from build123d import *

# Parameters (mm, degrees)
F0_R        = 2.35
F1_DEPTH    = 11.43
F0_R_2      = 4.636
F2_DEPTH    = 3.81
F0_R_3      = 11
F3_DEPTH    = 2.54
F5_DEPTH    = 1.27
F6_T1_DEPTH = 12.7
F6_T3_DEPTH = 7.62
F6_T5_DEPTH = 4.445
F6_T7_DEPTH = 4.079017898
F6_T9_DEPTH = 6.0188206533


# Not quite as in the source:
# - a fillet or chamfer that OpenCascade refuses, or shapes differently, is made with other operations: its cross-section is extruded or revolved along the edge and cut away or added


with BuildPart() as f1:
    # F0 (on Top) → F1 (new body)
    with BuildSketch(Plane.XY):
        Circle(F0_R)
    extrude(amount=F1_DEPTH)

    # F0 (on Top) → F2 (join)
    with BuildSketch(Plane.XY):
        Circle(F0_R_2)
        Circle(F0_R, mode=Mode.SUBTRACT)
    extrude(amount=F2_DEPTH)

    # F0 (on Top) → F3 (join)
    with BuildSketch(Plane.XY):
        Circle(F0_R_3)
        Circle(F0_R_2, mode=Mode.SUBTRACT)
    extrude(amount=F3_DEPTH)

    # F4 (on face) → F5 (join)
    with BuildSketch(Plane.XY):
        with BuildLine():
            ThreePointArc((0, -6.7733326328), (-6.1696334492, -0.6777773574), (0, 5.417777918))
            ThreePointArc((0, 5.417777918), (1.9417265012, 4.2834880284), (2.4694073737, 2.0975172472))
            Line((2.4694073737, 2.0975172472), (4.8922184175, 2.0975172472))
            ThreePointArc((4.8922184175, 2.0975172472), (3.5875761059, 5.9808584475), (0, 7.9586673672))
            ThreePointArc((0, 7.9586673672), (-8.382, -0.4233326328), (0, -8.8053326328))
            ThreePointArc((0, -8.8053326328), (3.39954986, -7.3527295439), (5.0117596984, -4.0259030648))
            Line((5.0117596984, -4.0259030648), (2.4717596984, -4.0259030648))
            ThreePointArc((2.4717596984, -4.0259030648), (1.8244333866, -5.9291174694), (0, -6.7733326328))
        make_face()
        with BuildLine():
            Line((4.8922184175, 2.0975172472), (2.4694073737, 2.0975172472))
            ThreePointArc((2.4694073737, 2.0975172472), (2.3960471942, 1.7747190007), (2.2859995271, 1.4625172472))
            Line((2.2859995271, 1.4625172472), (4.8259995271, 1.4625172472))
            ThreePointArc((4.8259995271, 1.4625172472), (4.8680955625, 1.7790801102), (4.8922184175, 2.0975172472))
        make_face()
        with BuildLine():
            ThreePointArc((2.2859995271, 1.4625172472), (2.3960471942, 1.7747190007), (2.4694073737, 2.0975172472))
            Line((2.4694073737, 2.0975172472), (0.3809995271, 2.0975172472))
            Line((0.3809995271, 2.0975172472), (0.3809995271, 0.8275172472))
            Line((0.3809995271, 0.8275172472), (6.7309995271, 0.8275172472))
            Line((6.7309995271, 0.8275172472), (6.7309995271, 2.0975172472))
            Line((6.7309995271, 2.0975172472), (4.8922184175, 2.0975172472))
            ThreePointArc((4.8922184175, 2.0975172472), (4.8680955625, 1.7790801102), (4.8259995271, 1.4625172472))
            Line((4.8259995271, 1.4625172472), (2.2859995271, 1.4625172472))
        make_face()
    extrude(amount=-F5_DEPTH)

    # F6: fillet of radius 1.27 on 5 edges, made by hand

    # F6_s2 → F6_t1 (cut)
    with BuildSketch(Plane.YZ.offset(-2.7940004729)):
        with BuildLine():
            ThreePointArc((0.8275172472, 0), (1.1994916351, -0.8980256121), (2.0975172472, -1.27))
            Line((2.0975172472, -1.27), (0.8275172472, -1.27))
            Line((0.8275172472, -1.27), (0.8275172472, 0))
        make_face()
    extrude(amount=F6_T1_DEPTH, mode=Mode.SUBTRACT)

    # F6_s4 → F6_t3 (cut)
    with BuildSketch(Plane.XZ.offset(-5.2725172472)):
        with BuildLine():
            ThreePointArc((6.7309995271, 0), (6.3590251392, -0.8980256121), (5.4609995271, -1.27))
            Line((5.4609995271, -1.27), (6.7309995271, -1.27))
            Line((6.7309995271, -1.27), (6.7309995271, 0))
        make_face()
    extrude(amount=F6_T3_DEPTH, mode=Mode.SUBTRACT)

    # F6_s6 → F6_t5 (cut)
    with BuildSketch(Plane.XZ.offset(-2.0975172472)):
        with BuildLine():
            ThreePointArc((0.3809995271, 0), (0.752973915, -0.8980256121), (1.6509995271, -1.27))
            Line((1.6509995271, -1.27), (0.3809995271, -1.27))
            Line((0.3809995271, -1.27), (0.3809995271, 0))
        make_face()
    extrude(amount=F6_T5_DEPTH, mode=Mode.SUBTRACT)

    # F6_s8 → F6_t7 (cut)
    with BuildSketch(Plane.XY.offset(-4.079017898)):
        with BuildLine():
            ThreePointArc((3.5953668576, -4.0259030648), (2.8338642738, -4.2795301928), (2.3765155692, -4.9391096556))
            ThreePointArc((2.3765155692, -4.9391096556), (2.4655394537, -4.4868244195), (2.4717596984, -4.0259030648))
            Line((2.4717596984, -4.0259030648), (3.5953668576, -4.0259030648))
        make_face()
    extrude(amount=F6_T7_DEPTH, mode=Mode.SUBTRACT)

    # F6_s10 → F6_t9 (cut)
    with BuildSketch(Plane.XY.offset(-6.0188206533)):
        with BuildLine():
            ThreePointArc((4.4971207542, -5.8543872382), (4.4340465678, -4.6237330343), (3.3565088886, -4.0259030648))
            Line((3.3565088886, -4.0259030648), (5.0117596984, -4.0259030648))
            ThreePointArc((5.0117596984, -4.0259030648), (4.837388646, -4.9634915319), (4.4971207542, -5.8543872382))
        make_face()
    extrude(amount=F6_T9_DEPTH, mode=Mode.SUBTRACT)


solid = f1.part
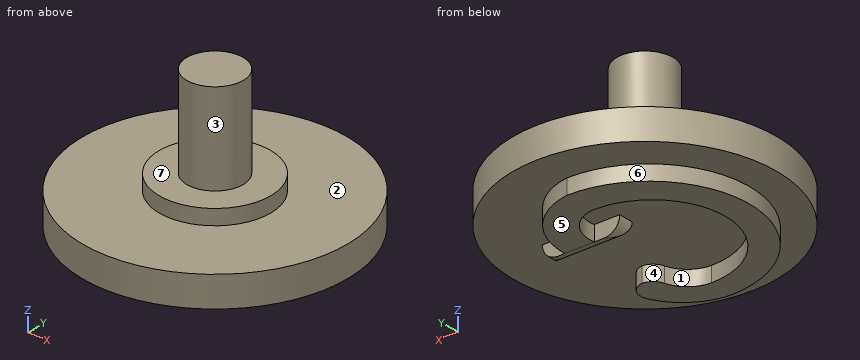
Could you check a few things on this model? Use its own coordinates, in mm. Face numbers are marked on the shaded views. A direction names the side the tool comes from. Give positions to 0.01 mm unless a question says otherwise; leave off trailing zeros. Loops run counter-clockwise (first coordinate to the right, second up) from the corner with the lowest first, then second, coordinate; pieces in that order, holes last. Notation, with made-up numbers: M -14.5,45.25 L -2.5,45.25 A11 cw -2.5,49.25 Z; hole C 62.5,55 d9. An arc over 180 degrees is marked long. Answer as a JSON object with one key per item and string values.
Q1. For the marked faces 4, 5, 6 and 7, which set-ups out of +Z, -Z, +X, -X, +Y, -Y let a thin tool reach every point of the face, with its end or its side?
Values found:
{"face 4": "-Z", "face 5": "-Z, +X, -X, +Y, -Y", "face 6": "-Z, -X", "face 7": "+Z"}
Q2. Suppose I cut it at A-A, the plane y = -7.5. List the corners of the cut face in (x, z) for me, plus the area to 3 significant figures.
Values found:
{"outline": "M -8.05,0 L -4.49,0 L -4.49,-1.27 L 3.24,-1.27 L 3.24,0 L 8.05,0 L 8.05,2.54 L -8.05,2.54 Z", "area": "50.7 mm²"}
Q3. Suppose I cut it at D-D, the plane y = 0. List the corners of the cut face in (x, z) for me, plus the area to 3 significant figures.
Values found:
{"outline": "M -11,0 L -8.37,0 L -8.37,-1.27 L -6.13,-1.27 L -6.13,0 L 11,0 L 11,2.54 L 4.64,2.54 L 4.64,3.81 L 2.35,3.81 L 2.35,11.43 L -2.35,11.43 L -2.35,3.81 L -4.64,3.81 L -4.64,2.54 L -11,2.54 Z", "area": "106 mm²"}
Q4. If we mould it in two halves opening along X, with no side actions, what happens to the marked faces 1, 2 and 3? For each: pulls with the +X half, pulls with the -X half, needs draft (parallel to the pull), parting line crosses it, or undercut.
Values found:
{"face 1": "undercut", "face 2": "needs draft", "face 3": "parting line crosses it"}
Q5. If I drill on probe 1 along Z at (x, y) = (-5.5, 7.75); probe 2 along Z at (x, y) = (-4.25, 5.5); probe 3 along X at (y, z) = (-9.5, 0.5), over which ranges is the centre line in solid material (lowest first)? Write a range as [from, to].
Values found:
{"probe 1": "z = [0, 2.54]", "probe 2": "z = [-1.27, 2.54]", "probe 3": "x = [-5.55, 5.55]"}
Q6. Suppose I cut it at C-C, the plane z = 7.75. List the corners of the cut face in (x, y) for me, plus the area to 3 significant figures.
Values found:
{"outline": "C 0,0 d4.7", "area": "17.3 mm²"}
Q7. For P1, Ø0.6, axis at x = 1, z = -0.5, coming from the +Y side; P2, Ø1.5, axis at x = -2.5, z = 0.5, coming from the +Y side; P3, Ø3, axis at x = -6.5, y = -0.5, coming from the +Z side, each with a flat end and sliding along its axis, tell me the tip position at first contact or that it passes through.
Values found:
{"P1": "stops at y = 7.82", "P2": "stops at y = 10.86", "P3": "stops at z = 2.54"}
Q8. Suppose I cut it at B-B, the plane x = -6.5. List the corners of the cut face in (y, z) for me.
Values found:
{"outline": "M -8.87,0 L -5.72,0 L -5.72,-1.27 L 4.87,-1.27 L 4.87,0 L 8.87,0 L 8.87,2.54 L -8.87,2.54 Z"}
